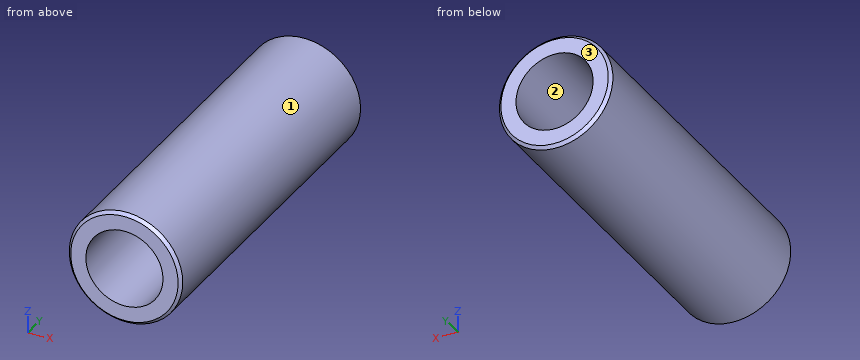
from build123d import *

# Parameters (mm, degrees)
SKETCH1_R           = 4.7625
BOSS_EXTRUDE1_DEPTH = 14.381250003
CHAMFER1_SIZE       = 0.254
SKETCH2_R           = 3.2385
CUT_EXTRUDE1_DEPTH  = 29.762500006


with BuildPart() as part:
    # Sketch1 → Boss-Extrude1 (new body, symmetric)
    with BuildSketch(Plane(origin=(0, 0, 0), x_dir=(1, 0, 0), z_dir=(0, 1, 0))):
        Circle(SKETCH1_R)
    extrude(amount=BOSS_EXTRUDE1_DEPTH, both=True)

    # Chamfer1
    chamfer1_edges = [part.edges().sort_by_distance(p)[0] for p in [
        (-4.7625, -14.381250003, 0),
        (-4.7625, 14.381250003, 0),
    ]]
    chamfer(chamfer1_edges, length=CHAMFER1_SIZE)

    # Sketch2 → Cut-Extrude1 (cut, through all)
    with BuildSketch(Plane.XZ.offset(14.381250003)):
        Circle(SKETCH2_R)
    extrude(amount=-CUT_EXTRUDE1_DEPTH, mode=Mode.SUBTRACT)


solid = part.part
Model file for the job. Use its own axes, mm. Face numbers are marked on the shaded views. Give positions to 0.01 mm unless a question says otherwise; leave off trailing zeros. Order: outer loops, then holes, each group sorted by start corner. A loop starts at its lowest first (then second) coordinate and runs counter-clockwise, first axis right, second up. Notation, with made-up numbers: (70.5, 70.5) - (109.5, 70.5) arc R30 cw to (109.5, 95.5) - close; hole circle Ø1 at (25.25, 11.25). An arc over 180 degrees is marked (long way). One line per item, written item: value.
Item 1: Slice it at C-C (y = -9.75). List the corners of the cut face in (x, z) (1 decimal).
Response values:
outline: circle Ø9.5 at (0, 0); hole circle Ø6.5 at (0, 0)
Item 2: Wall check: line 1 (Z direction, x = 0, y = 4.5); line 2 (Z direction, x = -2.75, y = 9.75); line 3 (X direction, y = -10.5, z = 0.75). Give the ranges that are in metal, low to high.
Response values:
line 1: -4.76 to -3.24, 3.24 to 4.76
line 2: -3.89 to -1.71, 1.71 to 3.89
line 3: -4.7 to -3.15, 3.15 to 4.7
Item 3: Slice it at B-B (z = 0). List the corners of the cut face in (x, y).
Response values:
outline: (-4.76, -14.13) - (-4.51, -14.38) - (-3.24, -14.38) - (-3.24, 14.38) - (-4.51, 14.38) - (-4.76, 14.13) - close; (3.24, -14.38) - (4.51, -14.38) - (4.76, -14.13) - (4.76, 14.13) - (4.51, 14.38) - (3.24, 14.38) - close
Item 4: Slice it at A-A (x = 0). List the corners of the cut face in (y, z).
Response values:
outline: (-14.38, -4.51) - (-14.13, -4.76) - (14.13, -4.76) - (14.38, -4.51) - (14.38, -3.24) - (-14.38, -3.24) - close; (-14.38, 3.24) - (14.38, 3.24) - (14.38, 4.51) - (14.13, 4.76) - (-14.13, 4.76) - (-14.38, 4.51) - close
Item 5: Two-plate mould, pull along X, no slides. Class the marked faces 1, 2 and 3: released by +X, released by -X, zero draft, split by the parting line, or undercut.
Response values:
face 1: split by the parting line
face 2: undercut
face 3: zero draft
